Source: CAD feature listing. Evaluate the final solid. Frame: model axes, mm. Face numbers are marked on the shaded views. A direction names the side the tool comes from. Round coordinates to 2 decimals unless told otherwise and drop trailing zeros. Write each loop counter-clockwise with the first axis right and the second up, starting at its lowest first coordinate (ties: lowest second). Pieces come first, ordered by that corner, then holes. Notation, with made-up numbers: (-13, -30) -> (25, -30) arc R33 cw to (25, -2) -> close; hole circle Ø2 at (88.25, -38.5). An arc over 180 degrees is marked (long way). Put each result on its own line as item: value.
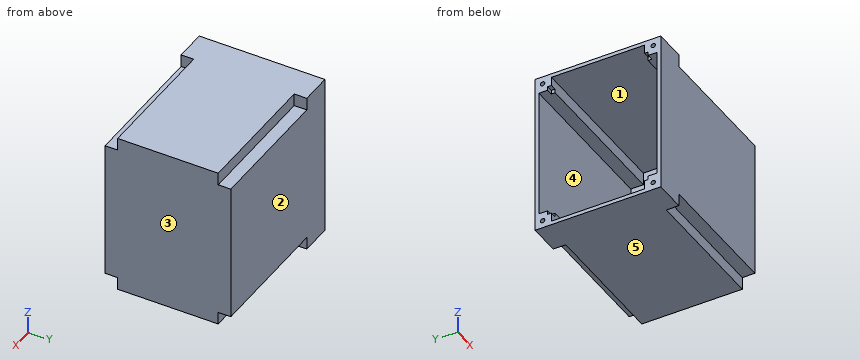
```python
from build123d import *

# Parameters (mm, degrees)
SKETCH2_W           = 130
SKETCH2_H           = 130
BOSS_EXTRUDE1_DEPTH = 100
SKETCH3_W           = 104
SKETCH3_H           = 74
CUT_EXTRUDE1_DEPTH  = 127
SKETCH4_W           = 10
SKETCH4_H           = 10
CUT_EXTRUDE3_DEPTH  = 105
SKETCH5_W           = 104
SKETCH5_H           = 10
CUT_EXTRUDE4_DEPTH  = 127
SKETCH6_W           = 10
SKETCH6_H           = 74
CUT_EXTRUDE5_DEPTH  = 127
SKETCH7_R           = 1.75
CUT_EXTRUDE6_DEPTH  = 20
SKETCH8_W           = 3
SKETCH8_H           = 3
CUT_EXTRUDE7_DEPTH  = 5


with BuildPart() as part:
    # Sketch2 → Boss-Extrude1 (new body)
    with BuildSketch(Plane(origin=(0, 0, 0), x_dir=(1, 0, 0), z_dir=(0, 1, 0))):
        with Locations((65, 65)):
            Rectangle(SKETCH2_W, SKETCH2_H)
    extrude(amount=BOSS_EXTRUDE1_DEPTH)

    # Sketch3 → Cut-Extrude1 (cut)
    with BuildSketch(Plane.ZY):
        with Locations((-65, 50)):
            Rectangle(SKETCH3_W, SKETCH3_H)
    extrude(amount=-CUT_EXTRUDE1_DEPTH, mode=Mode.SUBTRACT)

    # Sketch4 → Cut-Extrude3 (cut)
    with BuildSketch(Plane(origin=(130, 0, 0), x_dir=(0, 0, -1), z_dir=(1, 0, 0))):
        with Locations((5, 95)):
            Rectangle(SKETCH4_W, SKETCH4_H)
        with Locations((125, 95)):
            Rectangle(SKETCH4_W, SKETCH4_H)
        with Locations((5, 5)):
            Rectangle(SKETCH4_W, SKETCH4_H)
        with Locations((125, 5)):
            Rectangle(SKETCH4_W, SKETCH4_H)
    extrude(amount=-CUT_EXTRUDE3_DEPTH, mode=Mode.SUBTRACT)

    # Sketch5 → Cut-Extrude4 (cut)
    with BuildSketch(Plane.ZY):
        with Locations((-65, 92)):
            Rectangle(SKETCH5_W, SKETCH5_H)
        with Locations((-65, 8)):
            Rectangle(SKETCH5_W, SKETCH5_H)
    extrude(amount=-CUT_EXTRUDE4_DEPTH, mode=Mode.SUBTRACT)

    # Sketch6 → Cut-Extrude5 (cut)
    with BuildSketch(Plane.ZY):
        with Locations((-122, 50)):
            Rectangle(SKETCH6_W, SKETCH6_H)
        with Locations((-8, 50)):
            Rectangle(SKETCH6_W, SKETCH6_H)
    extrude(amount=-CUT_EXTRUDE5_DEPTH, mode=Mode.SUBTRACT)

    # Sketch7 → Cut-Extrude6 (cut)
    with BuildSketch(Plane.ZY):
        with Locations((-124, 94)):
            Circle(SKETCH7_R)
        with Locations((-6, 94)):
            Circle(SKETCH7_R)
        with Locations((-124, 6)):
            Circle(SKETCH7_R)
        with Locations((-6, 6)):
            Circle(SKETCH7_R)
    extrude(amount=-CUT_EXTRUDE6_DEPTH, mode=Mode.SUBTRACT)

    # Sketch8 → Cut-Extrude7 (cut)
    with BuildSketch(Plane.ZY):
        with Locations((-118.5, 88.5)):
            Rectangle(SKETCH8_W, SKETCH8_H)
        with Locations((-11.5, 88.5)):
            Rectangle(SKETCH8_W, SKETCH8_H)
        with Locations((-118.5, 11.5)):
            Rectangle(SKETCH8_W, SKETCH8_H)
        with Locations((-11.5, 11.5)):
            Rectangle(SKETCH8_W, SKETCH8_H)
    extrude(amount=-CUT_EXTRUDE7_DEPTH, mode=Mode.SUBTRACT)


solid = part.part
```
Q1. Draft query along Y for the marked faces 1, 2 and 3. Return one class per face: +Y half, -Y half, draft (parallel to the pull), parting line (faces both ways), or undercut.
Ans:
face 1: undercut
face 2: +Y half
face 3: draft
Q2. Pin query (flat end, axial travel): pin 1 (4.5 mm diameter, centred on y = 94, z = -6, fed in from +X); pin 2 (3 mm diameter, centred on x = 66.5, y = 93, fed in from +Z); pin 3 (2 mm diameter, centred on y = 26.5, z = -41.5, fed in from -X). Return the tip coordinate at first contact, or that it passes through.
Ans:
pin 1: stops at x = 25
pin 2: stops at z = -10
pin 3: stops at x = 127
Q3. Material intervals for line 1 (Z direction, x = 4.5, y = 94); line 2 (Y direction, x = 4, z = -6); line 3 (Z direction, x = 120.5, y = 39.5), sorted ascending. Write a range as [from, to].
Ans:
line 1: z = [-130, -125.75], [-122.25, -117], [-13, -7.75], [-4.25, 0]
line 2: y = [0, 4.25], [7.75, 13], [87, 92.25], [95.75, 100]
line 3: z = [-130, -127], [-3, 0]
Q4. Cut plane C-C on z = -33. Output: boundary loops of the cut face in (x, y).
Ans:
outline: (0, 0) -> (130, 0) -> (130, 100) -> (0, 100) -> (0, 97) -> (127, 97) -> (127, 3) -> (0, 3) -> close
Q5. Cut plane B-B on y = 94. Output: boundary loops of the cut face in (x, z).
Ans:
outline: (0, -130) -> (25, -130) -> (25, -120) -> (130, -120) -> (130, -10) -> (25, -10) -> (25, 0) -> (0, 0) -> (0, -4.25) -> (20, -4.25) -> (20, -7.75) -> (0, -7.75) -> (0, -13) -> (127, -13) -> (127, -117) -> (0, -117) -> (0, -122.25) -> (20, -122.25) -> (20, -125.75) -> (0, -125.75) -> close
Q6. Cut plane A-A on x = 121. Output: boundary loops of the cut face in (y, z), and give its area (3 significant figures).
Ans:
outline: (0, -120) -> (10, -120) -> (10, -130) -> (90, -130) -> (90, -120) -> (100, -120) -> (100, -10) -> (90, -10) -> (90, 0) -> (10, 0) -> (10, -10) -> (0, -10) -> close; hole (3, -117) -> (13, -117) -> (13, -127) -> (87, -127) -> (87, -117) -> (97, -117) -> (97, -13) -> (87, -13) -> (87, -3) -> (13, -3) -> (13, -13) -> (3, -13) -> close
area: 1,340 mm^2
Q7. Cut plane D-D on z = -6. Output: boundary loops of the cut face in (x, y).
Ans:
outline: (0, 0) -> (25, 0) -> (25, 10) -> (130, 10) -> (130, 90) -> (25, 90) -> (25, 100) -> (0, 100) -> (0, 95.75) -> (20, 95.75) -> (20, 92.25) -> (0, 92.25) -> (0, 87) -> (127, 87) -> (127, 13) -> (0, 13) -> (0, 7.75) -> (20, 7.75) -> (20, 4.25) -> (0, 4.25) -> close
Q8. Reachability of the marked faces 4 and 5 from +Z, -Z, +X, -X, +Y, -Y: full face, straight path, thin tool, end or side. Return the list, or none.
Ans:
face 4: -X
face 5: -Z, +X, -X, +Y, -Y
